Can you work these out from the model? Positions are in its coordinate system, mm. Face numbers are marked on the shaded views. A direction names the side the tool comes from. Round coordinates to 2 decimals unless told otherwise and drop trailing zeros. Write each loop counter-clockwise with the first axis right and the second up, starting at its lowest first coordinate (ties: lowest second). Pieces come first, ordered by that corner, then holes.
Q1. For the marked faces 1, 2 and 3, which set-ups out of +Z, -Z, +X, -X, +Y, -Y let a thin tool reach every point of the face, with its end or its side?
Q2. If we section it at B-B (x = 8.75): Please give me the cut outline in (y, z), plus the area to 3 significant figures.
Q3. We'd pull the mould along Y, two halves only. Please class the marked faces 4, 5 and 6: +Y half, -Y half, draft (parallel to the pull), parting line (faces both ways), or undercut.
Q4. If we section it at A-A (z = 15.25): Please give me the cut outline in (x, y).
Q5. If we section it at C-C (y = -7.75): Please give me the cut outline in (x, z), plus the area to 3 significant figures.
Q6. If we section it at D-D (z = 4.9): Please give me the cut outline in (x, y).
Q7. I'm going to push flat-ended pins straight in: pin 1 Ø6 at (y, z) = (0, -15.25) entering from +X; pin 2 Ø4 at (x, z) = (3, -5) entering from -Y; pin 3 Ø4 at (x, z) = (3.89, -4.9) entering from -Y. Where does each tip first touch, or does it pass through?
Q8. Please list where these lines run through material, in increasing order: line 1 along X through (y, z) = (-5, -4.9); line 2 along Y through (x, z) = (1.8, 15.25); line 3 along Z through (x, y) = (9, -1.25).
from build123d import *

# Parameters (mm, degrees)
SKETCH1_W           = 40.2
SKETCH1_H           = 20
BOSS_EXTRUDE1_DEPTH = 11.9
SKETCH2_R           = 2.35
CUT_EXTRUDE1_DEPTH  = 10
SKETCH3_R           = 2
CUT_EXTRUDE3_DEPTH  = 26.409053505
SKETCH5_R           = 3.25
CUT_EXTRUDE4_DEPTH  = 9
CHAMFER1_SIZE       = 1


with BuildPart() as part:
    # Sketch1 → Boss-Extrude1 (new body)
    with BuildSketch(Plane(origin=(0, 0, 0), x_dir=(0, 0, -1), z_dir=(1, 0, 0))):
        Rectangle(SKETCH1_W, SKETCH1_H)
    extrude(amount=BOSS_EXTRUDE1_DEPTH)

    # Sketch2 → Cut-Extrude1 (cut)
    with BuildSketch(Plane.XZ.offset(10)):
        with Locations(Location((3.89, -4.9, 0), (0, 0, 270))):
            Circle(SKETCH2_R)
        with Locations(Location((3.89, 4.9, 0), (0, 0, 90))):
            Circle(SKETCH2_R)
    extrude(amount=-CUT_EXTRUDE1_DEPTH, mode=Mode.SUBTRACT)

    # Sketch3 → Cut-Extrude3 (cut, through all)
    with BuildSketch(Plane(origin=(11.9, 0, 0), x_dir=(0, 0, -1), z_dir=(1, 0, 0))):
        with Locations((15.25, 0)):
            Circle(SKETCH3_R)
        with Locations(Location((-15.25, 0, 0), (0, 0, 180))):
            Circle(SKETCH3_R)
    extrude(amount=-CUT_EXTRUDE3_DEPTH, mode=Mode.SUBTRACT)

    # Sketch5 → Cut-Extrude4 (cut)
    with BuildSketch(Plane(origin=(11.9, 0, 0), x_dir=(0, 0, -1), z_dir=(1, 0, 0))):
        with Locations((15.25, 0)):
            Circle(SKETCH5_R)
        with Locations(Location((-15.25, 0, 0), (0, 0, 180))):
            Circle(SKETCH5_R)
    extrude(amount=-CUT_EXTRUDE4_DEPTH, mode=Mode.SUBTRACT)

    # Chamfer1
    chamfer1_edges = [part.edges().sort_by_distance(p)[0] for p in [
        (3.89, -10, -2.55),
        (3.89, -10, 2.55),
    ]]
    chamfer(chamfer1_edges, length=CHAMFER1_SIZE)


solid = part.part
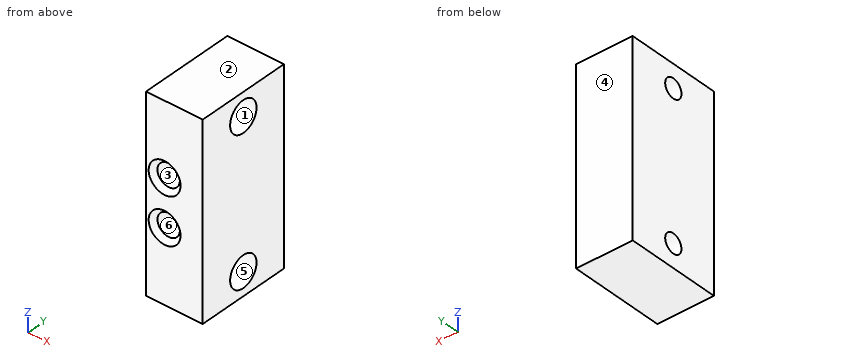
A:
1. face 1: +X
1. face 2: +Z, +X, -X, +Y, -Y
1. face 3: -Y
2. outline: (-10, -20.1) - (10, -20.1) - (10, 20.1) - (-10, 20.1) - close; hole circle Ø6.5 at (0, -15.25); hole circle Ø6.5 at (0, 15.25)
2. area: 738 mm2
3. face 4: +Y half
3. face 5: undercut
3. face 6: draft
4. outline: (0, -10) - (11.9, -10) - (11.9, -3.25) - (2.9, -3.25) - (2.9, -2) - (0, -2) - close; (0, 2) - (2.9, 2) - (2.9, 3.25) - (11.9, 3.25) - (11.9, 10) - (0, 10) - close
5. outline: (0, -20.1) - (11.9, -20.1) - (11.9, 20.1) - (0, 20.1) - close; hole circle Ø4.7 at (3.89, -4.9); hole circle Ø4.7 at (3.89, 4.9)
5. area: 444 mm2
6. outline: (0, -10) - (0.54, -10) - (1.54, -9) - (1.54, 0) - (6.24, 0) - (6.24, -9) - (7.24, -10) - (11.9, -10) - (11.9, 10) - (0, 10) - close
7. pin 1: stops at x = 2.9
7. pin 2: stops at y = -9.55
7. pin 3: stops at y = 0
8. line 1: x = 0 to 1.54, 6.24 to 11.9
8. line 2: y = -10 to -2, 2 to 10
8. line 3: z = -20.1 to -18.25, -12.25 to 12.25, 18.25 to 20.1
